CAD build for the part. Positions are in the model's coordinates, mm. Face numbers are marked on the shaded views. A direction names the side the tool comes from. Give positions to 0.01 mm unless a question says otherwise; leave off trailing zeros. Use one line per item in the form item = value. Start each with the question number.
from build123d import *

# Parameters (mm, degrees)
F0_W     = 31.75
F0_H     = 15.875
F0_R     = 2.38125
F1_DEPTH = 3.175
F2_DEPTH = 4.7625
F3_T     = -1.5875
F4_R     = 3.175
F4_R_2   = 2.38125
F5_DEPTH = 1.5875
F6_DEPTH = 6.35


with BuildPart() as f1:
    # F0 (on Top) → F1 (new body)
    with BuildSketch(Plane.XY):
        Rectangle(F0_W, F0_H)
        with Locations((-11.90625, -3.96875)):
            Circle(F0_R, mode=Mode.SUBTRACT)
        with Locations((-3.96875, -3.96875)):
            Circle(F0_R, mode=Mode.SUBTRACT)
        with Locations((3.96875, -3.96875)):
            Circle(F0_R, mode=Mode.SUBTRACT)
        with Locations((11.90625, -3.96875)):
            Circle(F0_R, mode=Mode.SUBTRACT)
        with Locations((-11.90625, 3.96875)):
            Circle(F0_R, mode=Mode.SUBTRACT)
        with Locations((-3.96875, 3.96875)):
            Circle(F0_R, mode=Mode.SUBTRACT)
        with Locations((3.96875, 3.96875)):
            Circle(F0_R, mode=Mode.SUBTRACT)
        with Locations((11.90625, 3.96875)):
            Circle(F0_R, mode=Mode.SUBTRACT)
    extrude(amount=F1_DEPTH)

    # F0 (on Top) → F2 (join)
    with BuildSketch(Plane.XY):
        with Locations((-11.90625, 3.96875)):
            Circle(F0_R)
        with Locations((-3.96875, 3.96875)):
            Circle(F0_R)
        with Locations((-3.96875, -3.96875)):
            Circle(F0_R)
        with Locations((-11.90625, -3.96875)):
            Circle(F0_R)
        with Locations((3.96875, 3.96875)):
            Circle(F0_R)
        with Locations((11.90625, 3.96875)):
            Circle(F0_R)
        with Locations((11.90625, -3.96875)):
            Circle(F0_R)
        with Locations((3.96875, -3.96875)):
            Circle(F0_R)
    extrude(amount=F2_DEPTH)

    # F3
    f3_openings = [f1.faces().sort_by_distance(p)[0] for p in [
        (0, 0, 0),
    ]]
    offset(amount=F3_T, openings=f3_openings, kind=Kind.INTERSECTION)

    # F4 (on face) → F5 (join)
    with BuildSketch(Plane(origin=(0, 0, 1.5875), x_dir=(1, 0, 0), z_dir=(0, 0, -1))):
        Circle(F4_R)
        Circle(F4_R_2, mode=Mode.SUBTRACT)
    extrude(amount=F5_DEPTH)

    # F6 (add): faces of the model
    f6_faces = [f1.faces().sort_by_distance(p)[0] for p in [
        (0, 7.5825242086, 0),
        (-3.0851974388, 0, 0),
    ]]
    extrude(f6_faces, amount=F6_DEPTH)


solid = f1.part
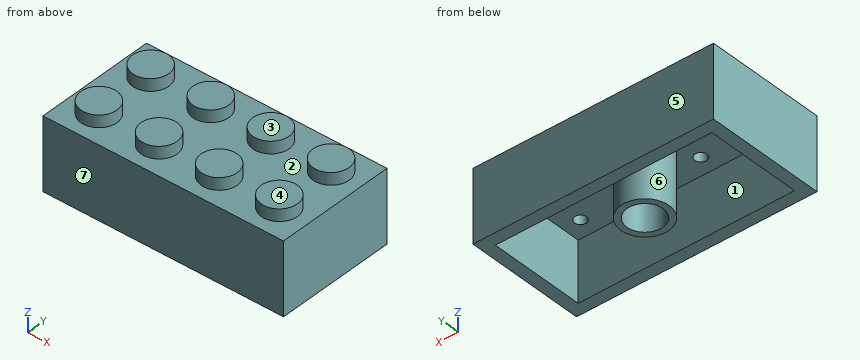
1) Pin check, flat tips, straight feed: pin 1 (0.5 mm diameter, centred on x = -12, y = 4, fed in from -Z) (3 decimals); pin 2 (5 mm diameter, centred on x = -6.5, y = 1.5, fed in from -Z). Stop position of each tip, or through.
2) 3-axis set-ups, long thin cutter, end or side, ignore diameter. For the marked faces 1, 2 and 3: which of +Z, -Z, +X, -X, +Y, -Y reach the whole face in a straight line?
3) Two-plate mould, pull along Y, no slides. Class the marked faces 4, 5, 6 and 7: released by +Y, released by -Y, zero draft, split by the parting line, or undercut.
4) Wall check: line 1 along X through (y, z) = (3.25, -1.25) (1 decimal); line 2 along Y through (x, z) = (-6.5, 0.5). Give the ranges that are in metal, low to high. Write a range as from..to.
5) Cut at A-A (z = 0). State how many separate pieces and enclosed holes the cut face has, and give its area (3 significant figures).
Final values:
q1.pin_1 = 3.175
q1.pin_2 = 1.59
q2.face_1 = -Z
q2.face_2 = +Z
q2.face_3 = +Z, +X, -X, +Y, -Y
q3.face_4 = zero draft
q3.face_5 = released by +Y
q3.face_6 = undercut
q3.face_7 = released by -Y
q4.line_1 = -15.9..-14.3, 14.3..15.9
q4.line_2 = -7.94..-6.35, 6.35..7.94
q5.separate_pieces = 2
q5.enclosed_holes = 2
q5.area = 155 mm^2
